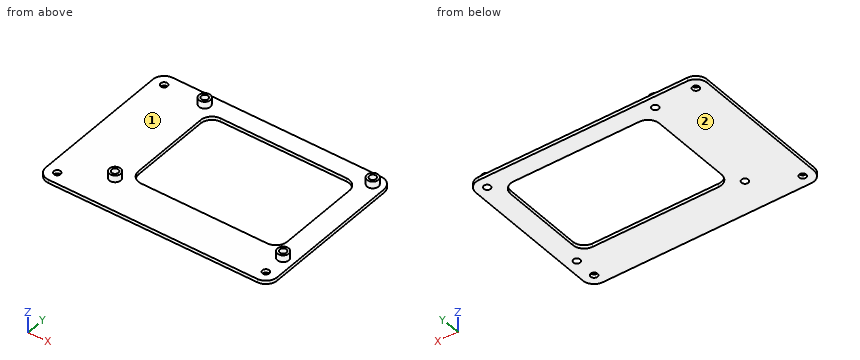
Autodesk Inventor part; units mm, degrees
ref_plane "YZ Plane" through (0, 0, 0) normal (1, 0, 0) x (0, 1, 0)
ref_plane "XZ Plane" through (0, 0, 0) normal (0, 1, 0) x (-1, 0, 0)
ref_plane "XY Plane" through (0, 0, 0) normal (0, 0, 1) x (1, 0, 0)
sketch "Sketch1" plane through (0, 0, 0) normal (0, 0, 1) x (1, 0, 0)
  line L0 (-37.05, 26) -> (37.05, 26) construction
  line L1 (37.05, 26) -> (37.05, -26) construction
  line L2 (37.05, -26) -> (-37.05, -26) construction
  line L3 (-37.05, -26) -> (-37.05, 26) construction
  line L4 (-37.05, 26) -> (37.05, -26) construction
  line L5 (37.05, 26) -> (-37.05, -26) construction
  circle A0 centre (37.05, 26) radius 1.5
  circle A1 centre (37.05, -26) radius 1.5
  circle A2 centre (-37.05, -26) radius 1.5
  circle A3 centre (-37.05, 26) radius 1.5
  line L6 (0, 45) -> (0, 0) construction
  line L7 (-18.2065, -55) -> (-18.2065, -15) construction
  circle A4 centre (37.05, 26) radius 3 construction
  circle A5 centre (37.05, -26) radius 3 construction
  circle A6 centre (-37.05, -26) radius 3 construction
  circle A7 centre (-37.05, 26) radius 3 construction
  line L8 (37.05, 26) -> (-54.95, 26) construction
  line L9 (-54.95, 26) -> (-54.95, -36) construction
  line L10 (-54.95, -36) -> (37.05, -36) construction
  line L11 (37.05, -36) -> (37.05, 26) construction
  circle A8 centre (-54.95, 26) radius 1.5
  circle A9 centre (-54.95, -36) radius 1.5
  circle A10 centre (37.05, -36) radius 1.5
  line L12 (-54.95, 31) -> (37.05, 31)
  line L13 (42.05, 26) -> (42.05, -36)
  line L14 (37.05, -41) -> (-54.95, -41)
  line L15 (-59.95, -36) -> (-59.95, 26)
  arc A11 (-54.95, 31) -> (-59.95, 26) centre (-54.95, 26) ccw
  arc A12 (-59.95, -36) -> (-54.95, -41) centre (-54.95, -36) ccw
  arc A13 (37.05, -41) -> (42.05, -36) centre (37.05, -36) ccw
  arc A14 (42.05, 26) -> (37.05, 31) centre (37.05, 26) ccw
  line L16 (27.775, -23) -> (-27.775, -23)
  line L17 (-32.775, -18) -> (-32.775, 18)
  line L18 (-27.775, 23) -> (27.775, 23)
  line L19 (32.775, 18) -> (32.775, -18)
  line L20 (32.775, -23) -> (-32.775, 23) construction
  line L21 (-32.775, -23) -> (32.775, 23) construction
  arc A15 (-27.775, 23) -> (-32.775, 18) centre (-27.775, 18) ccw
  arc A16 (32.775, 18) -> (27.775, 23) centre (27.775, 18) ccw
  arc A17 (27.775, -23) -> (32.775, -18) centre (27.775, -18) ccw
  arc A18 (-32.775, -18) -> (-27.775, -23) centre (-27.775, -18) ccw
  point P0 (0, 0)
  point P1 (0, 0)
  dimension "d0" = 74.1
  dimension "d1" = 52
  dimension "d2" = 3
  dimension "d3" = 45
  dimension "d4" = 6
  dimension "d5" = 0
  dimension "d8" = 62
  dimension "d9" = 92
  dimension "d10" = 5
  dimension "d11" = 5
  dimension "d12" = 5
  dimension "d13" = 5
  dimension "d14" = 5
  dimension "d15" = 5
  dimension "d16" = 3
extrude "Extrusion1" add sketch "Sketch1" along normal blind 1.5
sketch "Sketch2" plane through (0, 0, 1.5) normal (0, 0, 1) x (1, 0, 0)
  circle A0 centre (-37.05, 26) radius 1.5
  circle A1 centre (-37.05, 26) radius 2.5
  circle A2 centre (37.05, 26) radius 1.5
  circle A3 centre (37.05, 26) radius 2.5
  circle A4 centre (37.05, -26) radius 1.5
  circle A5 centre (37.05, -26) radius 2.5
  circle A6 centre (-37.05, -26) radius 1.5
  circle A7 centre (-37.05, -26) radius 2.5
  point P0 (0, 0)
  dimension "d19" = 5
extrude "Extrusion2" add sketch "Sketch2" along normal blind 3
properties part number "NewMoboAdapter"
Model file for the job. Use its own axes, mm. Face numbers are marked on the shaded views. Coordinates: 2 decimals unless noted, no trailing zeros. Order: outer loops, then holes, each group sorted by start corner. A loop starts at its lowest first (then second) coordinate and runs counter-clockwise, first axis right, second up. Notation, with made-up numbers: M 55.25,14.25 L 113.25,14.25 A14 ccw 113.25,20.25 Z; hole C 87,23.25 d8. An arc over 180 degrees is marked long. Return JSON: item names as keys, results as strings.
1. Saw through at C-C (x = -37.05). Give the cut face in (y, z), and give its area (3 significant figures).
Ans:
{"outline": "M -41,0 L -27.5,0 L -27.5,4.5 L -28.5,4.5 L -28.5,1.5 L -41,1.5 Z; M -24.5,0 L 24.5,0 L 24.5,4.5 L 23.5,4.5 L 23.5,1.5 L -23.5,1.5 L -23.5,4.5 L -24.5,4.5 Z; M 27.5,0 L 31,0 L 31,1.5 L 28.5,1.5 L 28.5,4.5 L 27.5,4.5 Z", "area": "111 mm^2"}
2. Saw through at B-B (y = -26). Give the cut face in (x, z), and give its area (3 significant figures).
Ans:
{"outline": "M -59.95,0 L -38.55,0 L -38.55,4.5 L -39.55,4.5 L -39.55,1.5 L -59.95,1.5 Z; M -35.55,0 L 35.55,0 L 35.55,4.5 L 34.55,4.5 L 34.55,1.5 L -34.55,1.5 L -34.55,4.5 L -35.55,4.5 Z; M 38.55,0 L 42.05,0 L 42.05,1.5 L 39.55,1.5 L 39.55,4.5 L 38.55,4.5 Z", "area": "156 mm^2"}
3. Flat gauge pin, fed straight in: pin 1 (1.5 mm diameter, centred on x = -27.5, y = -23.5, fed in from +Z). Where does the tip first touch, or does it go through?
Ans:
{"pin 1": "z = 1.5"}
4. Saw through at D-D (y = 0). Give the cut face in (x, z) (3 decimals), and give its area (3 significant figures).
Ans:
{"outline": "M -59.95,0 L -32.775,0 L -32.775,1.5 L -59.95,1.5 Z; M 32.775,0 L 42.05,0 L 42.05,1.5 L 32.775,1.5 Z", "area": "54.7 mm^2"}
5. Saw through at A-A (z = 2.75). Give the cut face in (x, y), and give its area (3 significant figures).
Ans:
{"outline": "C -37.05,-26 d5; C -37.05,26 d5; C 37.05,-26 d5; C 37.05,26 d5; hole C -37.05,-26 d3; hole C -37.05,26 d3; hole C 37.05,-26 d3; hole C 37.05,26 d3", "area": "50.3 mm^2"}
6. Drill centre lines: probe 1 along Y at (x, z) = (-54.95, 1.1); probe 2 along Y at (x, z) = (37.05, 2.85); probe 3 along X at (y, z) = (-17.5, 0.2) (3 decimals). Where is each one in solid material? Low to high.
Ans:
{"probe 1": "-41 to -37.5, -34.5 to 24.5, 27.5 to 31", "probe 2": "-28.5 to -27.5, -24.5 to -23.5, 23.5 to 24.5, 27.5 to 28.5", "probe 3": "-59.95 to -32.775, 32.775 to 42.05"}
7. Pull direction X, two halves, no side cores. Call the marked faces 1 and 2: +X half, -X half, draft (parallel to the pull), parting line (faces both ways), or undercut.
Ans:
{"face 1": "undercut", "face 2": "draft"}
